```python
from build123d import *

# Parameters (mm, degrees)
CROQUIS1_W              = 42
CROQUIS1_H              = 42
SALIENTE_EXTRUIR1_DEPTH = 38
CROQUIS2_R              = 11
SALIENTE_EXTRUIR2_DEPTH = 2
CROQUIS3_R              = 2.5
SALIENTE_EXTRUIR3_DEPTH = 13
CHAFL_N1_SIZE           = 4
CROQUIS4_R              = 1.5
CORTAR_EXTRUIR1_DEPTH   = 49.228622207
SALIENTE_EXTRUIR4_DEPTH = 3


with BuildPart() as part:
    # Croquis1 → Saliente-Extruir1 (new body)
    with BuildSketch(Plane.XY):
        Rectangle(CROQUIS1_W, CROQUIS1_H)
    extrude(amount=SALIENTE_EXTRUIR1_DEPTH)

    # Croquis2 → Saliente-Extruir2 (add)
    with BuildSketch(Plane.XY.offset(38)):
        Circle(CROQUIS2_R)
    extrude(amount=SALIENTE_EXTRUIR2_DEPTH)

    # Croquis3 → Saliente-Extruir3 (add)
    with BuildSketch(Plane.XY.offset(40)):
        with Locations(Location((0, 0, 0), (0, 0, 180))):
            Circle(CROQUIS3_R)
    extrude(amount=SALIENTE_EXTRUIR3_DEPTH)

    # Chaflán1
    chafl_n1_edges = [part.edges().sort_by_distance(p)[0] for p in [
        (21, -21, 19),
        (-21, -21, 19),
        (-21, 21, 19),
        (21, 21, 19),
    ]]
    chamfer(chafl_n1_edges, length=CHAFL_N1_SIZE)

    # Croquis4 → Cortar-Extruir1 (cut, through all)
    with BuildSketch(Plane.XY.offset(38)):
        with Locations((15.5, 15.5)):
            Circle(CROQUIS4_R)
        with Locations((-15.5, 15.5)):
            Circle(CROQUIS4_R)
        with Locations((-15.5, -15.5)):
            Circle(CROQUIS4_R)
        with Locations((15.5, -15.5)):
            Circle(CROQUIS4_R)
    extrude(amount=-CORTAR_EXTRUIR1_DEPTH, mode=Mode.SUBTRACT)

    # Croquis6 → Saliente-Extruir4 (add)
    with BuildSketch(Plane.XZ.offset(21)):
        with BuildLine():
            Line((1.353116467, 3.113624341), (-1.353116467, 3.113624341))
            ThreePointArc((-1.353116467, 3.113624341), (-2.014015037, 3.77452291), (-1.353116467, 4.43542148))
            Line((-1.353116467, 4.43542148), (1.353116467, 4.43542148))
            ThreePointArc((1.353116467, 4.43542148), (2.014015037, 3.77452291), (1.353116467, 3.113624341))
        make_face()
    extrude(amount=SALIENTE_EXTRUIR4_DEPTH)


solid = part.part
```
Build history of the part. All positions in model axes, mm. A direction names the side the tool comes from. Give positions to 0.01 mm unless a question says otherwise; leave off trailing zeros. Loops run counter-clockwise (first coordinate to the right, second up) from the corner with the lowest first, then second, coordinate; pieces in that order, holes last.
1) Band-saw the part on A-A on y = -15.5. List the corners of the cut face in (x, z).
Values follow:
outline: (-21, 0) - (-17, 0) - (-17, 38) - (-21, 38) - close; (-14, 0) - (14, 0) - (14, 38) - (-14, 38) - close; (17, 0) - (21, 0) - (21, 38) - (17, 38) - close
2) 3-axis set-ups, long thin cutter, end or side, ignore diameter. For faces 1 (the face through (0, -22, 4.435)), 2 (the face through (0, -22, 3.114)), 3 (the face through (-10, 10, 38)): which of +Z, -Z, +X, -X, +Y, -Y reach the whole face in a straight line?
Values follow:
face 1: +Z, +X, -X, -Y
face 2: -Z, +X, -X, -Y
face 3: +Z
3) Band-saw the part on C-C on z = 14. List the corners of the cut face in (x, y).
Values follow:
outline: (-21, -17) - (-17, -21) - (17, -21) - (21, -17) - (21, 17) - (17, 21) - (-17, 21) - (-21, 17) - close; hole circle Ø3 at (-15.5, -15.5); hole circle Ø3 at (-15.5, 15.5); hole circle Ø3 at (15.5, -15.5); hole circle Ø3 at (15.5, 15.5)
4) Band-saw the part on D-D on y = 0. List the corners of the cut face in (x, z), then the cut area to 4 significant figures.
Values follow:
outline: (-21, 0) - (21, 0) - (21, 38) - (11, 38) - (11, 40) - (2.5, 40) - (2.5, 53) - (-2.5, 53) - (-2.5, 40) - (-11, 40) - (-11, 38) - (-21, 38) - close
area: 1,705 mm2
5) Two-plate mould, pull along X, no slides. Class faces 4 (the face through (0, -24, 4)), 5 (the face through (-19, -19, 19)), 6 (the face through (2.014, -22.479, 3.789)), 7 (the face through (14, -15.43, 19.27)): released by +X, released by -X, zero draft, split by the parting line, or undercut.
Values follow:
face 4: zero draft
face 5: released by -X
face 6: released by +X
face 7: undercut
6) Probe line 1 along Y through (x, z) = (-15.5, 17.5); line 2 along Y through (x, z) = (15, 18). List the from-to ranges inside material, lowest first.
Values follow:
line 1: y = -21 to -17, -14 to 14, 17 to 21
line 2: y = -21 to -16.91, -14.09 to 14.09, 16.91 to 21
7) Drop flat-ended pins along their axis: P1, Ø4, axis at x = -15.5, y = 15.5, coming from the +Z side; P2, Ø1, axis at x = -4, z = 26, coming from the -Y side; P3, Ø2, axis at x = 0.5, y = -23, coming from the -Z side. Give the stop position or say it passes through.
Values follow:
P1: stops at z = 38
P2: stops at y = -21
P3: stops at z = 3.11
